```python
from build123d import *

# Parameters (mm, degrees)
SKETCH1_R           = 2
BOSS_EXTRUDE1_DEPTH = 400


with BuildPart() as part:
    # Sketch1 → Boss-Extrude1 (new body)
    with BuildSketch(Plane.XY):
        Polygon((-10, -20), (-3.5, -20), (-3.5, -19), (-3, -19), (-3, -18), (-5.5, -18), (-5.5, -16.560660172), (-3.44, -14.500660172), (3.44, -14.500660172), (5.5, -16.560660172), (5.5, -18), (3, -18), (3, -19), (3.5, -19), (3.5, -20), (10, -20), (10, -13.5), (9, -13.5), (9, -13), (8, -13), (8, -15.5), (6.560660172, -15.5), (4.500660172, -13.44), (4.500660172, -6.56), (6.560660172, -4.5), (8, -4.5), (8, -7), (9, -7), (9, -6.5), (10, -6.5), (10, 6.5), (9, 6.5), (9, 7), (8, 7), (8, 4.5), (6.560660172, 4.5), (4.500660172, 6.56), (4.500660172, 13.44), (6.560660172, 15.5), (8, 15.5), (8, 13), (9, 13), (9, 13.5), (10, 13.5), (10, 20), (3.5, 20), (3.5, 19), (3, 19), (3, 18), (5.5, 18), (5.5, 16.560660172), (3.44, 14.500660172), (-3.44, 14.500660172), (-5.5, 16.560660172), (-5.5, 18), (-3, 18), (-3, 19), (-3.5, 19), (-3.5, 20), (-10, 20), (-10, 13.5), (-9, 13.5), (-9, 13), (-8, 13), (-8, 15.5), (-6.560660172, 15.5), (-4.500660172, 13.44), (-4.500660172, 6.56), (-6.560660172, 4.5), (-8, 4.5), (-8, 7), (-9, 7), (-9, 6.5), (-10, 6.5), (-10, -6.5), (-9, -6.5), (-9, -7), (-8, -7), (-8, -4.5), (-6.560660172, -4.5), (-4.500660172, -6.56), (-4.500660172, -13.44), (-6.560660172, -15.5), (-8, -15.5), (-8, -13), (-9, -13), (-9, -13.5), (-10, -13.5), align=None)
        with Locations((0, 10)):
            Circle(SKETCH1_R, mode=Mode.SUBTRACT)
        with Locations((0, -10)):
            Circle(SKETCH1_R, mode=Mode.SUBTRACT)
        Polygon((-4.439339828, 4.5), (4.439339828, 4.5), (6.103256126, 2.836083702), (8, 2.836083702), (8, -2.999669914), (5.939669914, -2.999669914), (4.44, -4.499339828), (-4.44, -4.499339828), (-5.939669914, -2.999669914), (-8, -2.999669914), (-8, 3.000330086), (-5.939009742, 3.000330086), align=None, mode=Mode.SUBTRACT)
    extrude(amount=BOSS_EXTRUDE1_DEPTH)


solid = part.part
```
For this review, take the finished solid that the model builds, in its own axes (mm). Give positions to 0.01 mm unless a question says otherwise; leave off trailing zeros. Answer as a JSON object with one key per item and string values. Group by question number.
Item 1: For pin 1 Ø10 at (x, z) = (-3, 221.5) entering from -Y; pin 2 Ø1.5 at (y, z) = (9, 258) entering from +X; pin 3 Ø0.6 at (y, z) = (-13, 294) entering from +X, all flat-tipped, find the tip position at first contact; note any pin that passes through.
Item 2: For probe 1 along Y at (x, z) = (0, 246); probe 2 along Y at (x, z) = (8.75, 65); probe 3 along Y at (x, z) = (-0.5, 212), list the stretches that pass through material, from the lowest coordinate up. Write a range as [from, to].
Item 3: Draft analysis for pull direction Y (two halves, no side actions). For faces 1 (the flat face through (7, 20, 197)), 2 (the flat face through (4.501, -10, 197)), 3 (the flat face through (0, 5, 400)), state which applies: +Y half, -Y half, draft (parallel to the pull), parting line (faces both ways), or undercut.
Item 4: Consider section A-A on z = 345.5. Count the separate pieces of the cut face and the enclosed holes in it, plus the area to 3 significant figures.
Check result:
{
 "1": {"pin 1": "stops at y = -20", "pin 2": "stops at x = 4.5", "pin 3": "stops at x = 9"},
 "2": {"probe 1": "y = [-14.5, -12], [-8, -4.5], [4.5, 8], [12, 14.5]", "probe 2": "y = [-20, -13], [-7, 7], [13, 20]", "probe 3": "y = [-14.5, -11.94], [-8.06, -4.5], [4.5, 8.06], [11.94, 14.5]"},
 "3": {"face 1": "+Y half", "face 2": "undercut", "face 3": "draft"},
 "4": {"separate pieces": "1", "enclosed holes": "3", "area": "365 mm^2"}
}
